Drawing for the job (mm, zero at the part's lowest x, y, z). A direction names the side the tool comes from. Round coordinates to 2 decimals unless told otherwise and drop trailing zeros. Order: outer loops, then holes, each group sorted by start corner. A loop starts at its lowest first (then second) coordinate and runs counter-clockwise, first axis right, second up. Notation, with made-up numbers: (-16.75, 16.5) - (12.25, 16.5) arc R18 ccw to (12.25, 50.5) - close; hole circle Ø5 at (74, 68). An arc over 180 degrees is marked (long way). Answer as a JSON object with one key per item and string values.
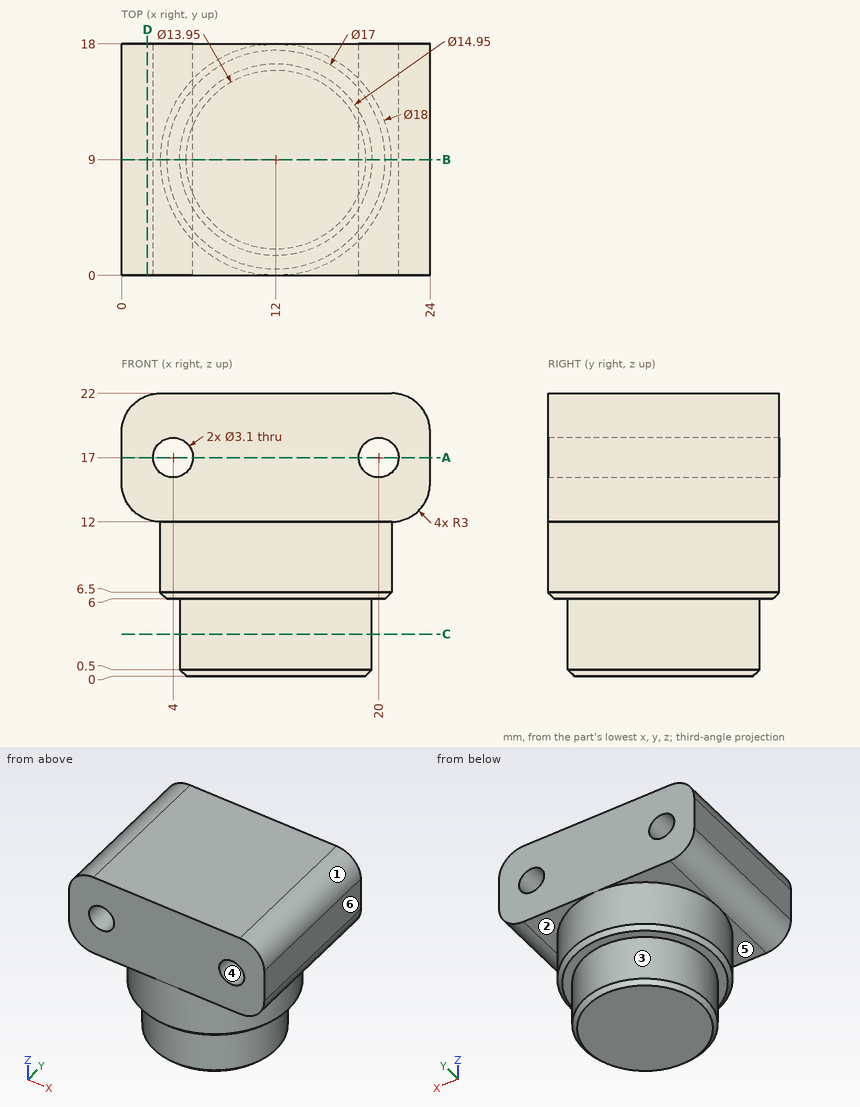
Item 1: Cut at C-C (z = 3.25). Write the cut outline in (x, y) (3 decimals).
Taken from the geometry:
{"outline": "circle Ø14.95 at (12, 9)"}
Item 2: Drop flat-ended pins along their axis: P1, Ø4, axis at y = 13.5, z = 13.5, coming from the -X side; P2, Ø8, axis at y = 13, z = 7, coming from the +X side; P3, Ø3, axis at x = 15, z = 7.5, coming from the +Y side. Give the stop position or say it passes through.
Taken from the geometry:
{"P1": "x = 0", "P2": "x = 21", "P3": "y = 17.87"}
Item 3: Cut at A-A (z = 17). Write the cut outline in (x, y), plus the area to 3 significant figures.
Taken from the geometry:
{"outline": "(0, 0) - (2.45, 0) - (2.45, 18) - (0, 18) - close; (5.55, 0) - (18.45, 0) - (18.45, 18) - (5.55, 18) - close; (21.55, 0) - (24, 0) - (24, 18) - (21.55, 18) - close", "area": "320 mm2"}
Item 4: Probe L1, parallel to X at y = 10, z = 17; L2, parallel to X at y = 13.25, z = 17.75; L3, parallel to Z at x = 5.75, y = 4.25. List the from-to ranges inside material, lowest first. Write a range as from..to.
Taken from the geometry:
{"L1": "0..2.45, 5.55..18.45, 21.55..24", "L2": "0..2.64, 5.36..18.64, 21.36..24", "L3": "6..22"}
Item 5: Cut at B-B (y = 9). State how many separate pieces and enclosed holes the cut face has, plus the area to 3 significant figures.
Taken from the geometry:
{"separate pieces": "1", "enclosed holes": "2", "area": "414 mm2"}
Item 6: Two-plate mould, pull along Z, no slides. Class the marked faces 4, 5 and 6: pulls with the +Z half, pulls with the -Z half, needs draft (parallel to the pull), parting line crosses it, or undercut.
Taken from the geometry:
{"face 4": "undercut", "face 5": "pulls with the -Z half", "face 6": "needs draft"}
Item 7: Tool access for the marked faces 1, 2 and 3: list every direction of +Z, -Z, +X, -X, +Y, -Y with a clear straight run to the whole face (end or side of a thin tool).
Taken from the geometry:
{"face 1": "+Z, +X, +Y, -Y", "face 2": "-Z, +X", "face 3": "-Z"}
Item 8: Cut at D-D (x = 2). Write the cut outline in (y, z).
Taken from the geometry:
{"outline": "(0, 12.17) - (18, 12.17) - (18, 21.83) - (0, 21.83) - close"}
